Design review of the part built by this model. Coordinates are the model's own, in mm. Face numbers are marked on the shaded views. A direction names the side the tool comes from. Round coordinates to 2 decimals unless told otherwise and drop trailing zeros. Order: outer loops, then holes, each group sorted by start corner. A loop starts at its lowest first (then second) coordinate and runs counter-clockwise, first axis right, second up. Notation, with made-up numbers: M 10.25,-36.75 L 31.25,-36.75 A6 cw 31.25,-28.75 Z; hole C 47,-7.5 d8. An arc over 180 degrees is marked long. Use a Markdown table: item, result. Add a question column.
(1) Take a section at A-A (z = 0). Write out the cut boundary in (x, y), then the cut area to 3 significant figures.
(2) Machinability: for the marked faces 1 and 2, which of the approach directions +Z, -Z, +X, -X, +Y, -Y give a long, thin tool a straight path to every point of the face, cutting with its end or side? Answer none if there is none.
(3) For pin 1 (3 mm diameter, centred on x = -2, y = 7, fed in from -Z); pin 2 (4.5 mm diameter, centred on x = 7.42, z = -7.42, fed in from +Y); pin 3 (3 mm diameter, centred on x = 4.5, z = -9.5, fed in from -Y), all flat-tipped, find the tip position at first contact; note any pin that passes through.
(4) Take a section at C-C (y = 18.5). Write out the cut boundary in (x, z).
(5) Take a section at B-B (x = 0). Write out the cut boundary in (y, z).
(6) Take a section at D-D (z = -8.25). Write out the cut boundary in (x, y), then the cut area to 3 significant figures.
(7) To check wall thickness, follow probe 1 along Y at (x, z) = (5.5, -5.5); probe 2 along Y at (x, z) = (0, 14); probe 3 along Z at (x, y) = (3.5, 9.5). State the ranges of each line that lie inside material, in increasing order. Write a range as from..to.
```python
from build123d import *

# Parameters (mm, degrees)
SKETCH1_W           = 26
SKETCH1_H           = 30
BOSS_EXTRUDE1_DEPTH = 1.5
BOSS_EXTRUDE2_DEPTH = 1.5
SKETCH4_R           = 4
CUT_EXTRUDE1_DEPTH  = 47.100433837
FILLET1_R           = 1
FILLET2_R           = 2
SKETCH5_R           = 5
SKETCH5_R_2         = 2
CUT_EXTRUDE2_DEPTH  = 39.082148049


with BuildPart() as part:
    # Sketch1 → Boss-Extrude1 (new body)
    with BuildSketch(Plane(origin=(0, 0, 0), x_dir=(1, 0, 0), z_dir=(0, 1, 0))):
        Rectangle(SKETCH1_W, SKETCH1_H)
    extrude(amount=BOSS_EXTRUDE1_DEPTH)

    # Sketch3 → Boss-Extrude2 (add)
    with BuildSketch(Plane.XY.offset(15)):
        with BuildLine():
            Line((-13, 1.5), (-13, 19.5))
            ThreePointArc((-13, 19.5), (0, 32.5), (13, 19.5))
            Line((13, 19.5), (13, 1.5))
            Line((13, 1.5), (-13, 1.5))
        make_face()
    extrude(amount=-BOSS_EXTRUDE2_DEPTH)

    # Sketch4 → Cut-Extrude1 (cut, through all)
    with BuildSketch(Plane.XY.offset(15)):
        with Locations((0, 19.5)):
            Circle(SKETCH4_R)
    extrude(amount=-CUT_EXTRUDE1_DEPTH, mode=Mode.SUBTRACT)

    # Fillet1
    fillet1_edges = [part.edges().sort_by_distance(p)[0] for p in [
        (0, 1.5, 13.5),
        (0, 0, 15),
    ]]
    fillet(fillet1_edges, radius=FILLET1_R)

    # Fillet2
    fillet2_edges = [part.edges().sort_by_distance(p)[0] for p in [
        (-13, 0.75, -15),
        (13, 0.75, -15),
    ]]
    fillet(fillet2_edges, radius=FILLET2_R)

    # Sketch5 → Cut-Extrude2 (cut, through all)
    with BuildSketch(Plane.XZ):
        with Locations(Location((0, 0, 0), (0, 0, 270))):
            Circle(SKETCH5_R)
        with Locations(Location((7.424621202, 7.424621202, 0), (0, 0, 270))):
            Circle(SKETCH5_R_2)
        with Locations(Location((-7.424621202, -7.424621202, 0), (0, 0, 270))):
            Circle(SKETCH5_R_2)
        with Locations(Location((-7.424621202, 7.424621202, 0), (0, 0, 270))):
            Circle(SKETCH5_R_2)
        with Locations(Location((7.424621202, -7.424621202, 0), (0, 0, 270))):
            Circle(SKETCH5_R_2)
    extrude(amount=-CUT_EXTRUDE2_DEPTH, mode=Mode.SUBTRACT)


solid = part.part
```
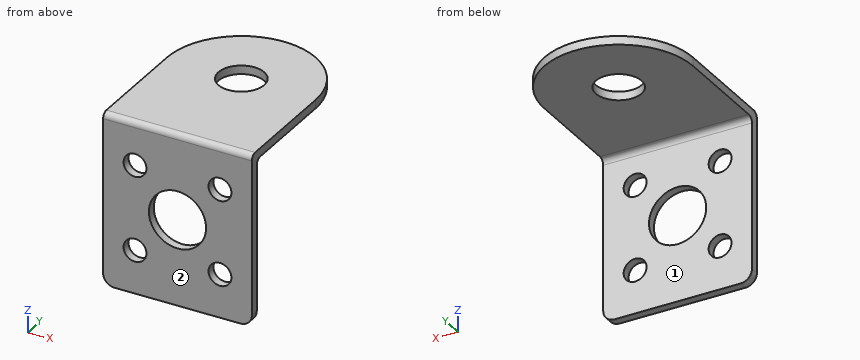
Verdict:
| question | item | result |
|---|---|---|
| 1 | outline | M -13,0 L -5,0 L -5,1.5 L -13,1.5 Z; M 5,0 L 13,0 L 13,1.5 L 5,1.5 Z |
| 1 | area | 24.0 mm^2 |
| 2 | face 1 | -Z, +X, -X, +Y |
| 2 | face 2 | +Z, -Z, +X, -X, -Y |
| 3 | pin 1 | stops at z = 13.5 |
| 3 | pin 2 | stops at y = 1.5 |
| 3 | pin 3 | stops at y = 0 |
| 4 | outline | M -13,13.5 L -3.87,13.5 L -3.87,15 L -13,15 Z; M 3.87,13.5 L 13,13.5 L 13,15 L 3.87,15 Z |
| 5 | outline | M 0,-15 L 1.5,-15 L 1.5,-5 L 0,-5 Z; M 0,5 L 1.5,5 L 1.5,12.5 A1 cw 2.5,13.5 L 15.5,13.5 L 15.5,15 L 1,15 A1 ccw 0,14 Z; M 23.5,13.5 L 32.5,13.5 L 32.5,15 L 23.5,15 Z |
| 6 | outline | M -13,0 L -9.25,0 L -9.25,1.5 L -13,1.5 Z; M -5.6,0 L 5.6,0 L 5.6,1.5 L -5.6,1.5 Z; M 9.25,0 L 13,0 L 13,1.5 L 9.25,1.5 Z |
| 6 | area | 28.1 mm^2 |
| 7 | probe 1 | y = 0..1.5 |
| 7 | probe 2 | y = 0..15.5, 23.5..32.5 |
| 7 | probe 3 | z = 13.5..15 |
